Geometry check sheet. Reference: the model listing, model coordinates, mm. Coordinates: 2 decimals unless noted, no trailing zeros. Loops run counter-clockwise (first coordinate to the right, second up) from the corner with the lowest first, then second, coordinate; pieces in that order, holes last. Notation, with made-up numbers: (84.25, 63) - (117.25, 63) arc R19 ccw to (117.25, 73) - close; hole circle Ø4 at (68.25, 70.5). An arc over 180 degrees is marked (long way). One line per item, written item: value.
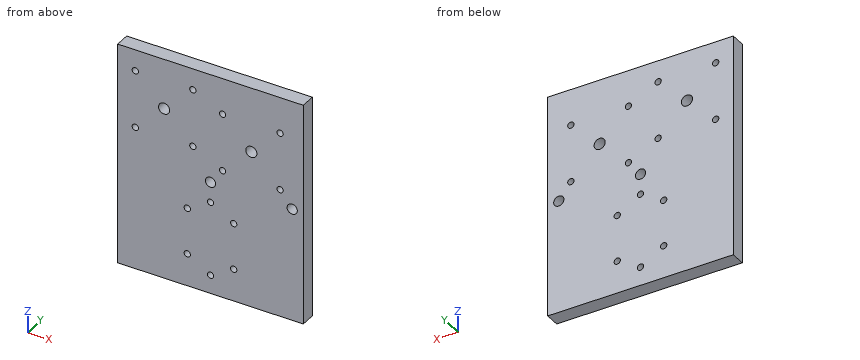
Autodesk Inventor part; units mm, degrees
ref_plane "YZ Plane" through (0, 0, 0) normal (1, 0, 0) x (0, 1, 0)
ref_plane "XZ Plane" through (0, 0, 0) normal (0, 1, 0) x (-1, 0, 0)
ref_plane "XY Plane" through (0, 0, 0) normal (0, 0, 1) x (1, 0, 0)
sketch "Skizze1" plane through (0, 0, 0) normal (0, 1, 0) x (-1, 0, 0)
  line L0 (50, -60) -> (-50, -60)
  line L1 (-50, -60) -> (-50, 60)
  line L2 (-50, 60) -> (50, 60)
  line L3 (50, 60) -> (50, -60)
  line L4 (50, -60) -> (-50, 60) construction
  line L5 (-50, -60) -> (50, 60) construction
  point P0 (0, 0)
  dimension "d0" = 100
  dimension "d1" = 120
extrude "Extrusion1" add sketch "Skizze1" along normal blind 8
sketch "Skizze2" plane through (0, 8, 0) normal (0, 1, 0) x (1, 0, 0)
  line L0 (-50, -60) -> (50, -60)
  line L1 (0, -60) -> (0, 152.9688)
  line L2 (50, 60) -> (-50, 60)
  point P0 (0, 0)
  point P1 (0, 10)
  point P2 (0, 50)
  dimension "d4" = 40
  dimension "d5" = 10
hole "Rail_through_holes" at (0, 8, -10) at (0, 8, -50) direction (0, -1, 0) diameter 3.4 end through all
sketch "Skizze3" plane through (0, 8, 0) normal (0, 1, 0) x (1, 0, 0)
  line L0 (-50, -60) -> (50, -60)
  line L1 (0, -60) -> (0, 60)
  line L2 (50, 60) -> (-50, 60)
  line L3 (12.5, 17.5) -> (-12.5, 17.5) construction
  line L4 (-12.5, 17.5) -> (-12.5, 42.5) construction
  line L5 (-12.5, 42.5) -> (12.5, 42.5) construction
  line L6 (12.5, 42.5) -> (12.5, 17.5) construction
  line L7 (12.5, 17.5) -> (-12.5, 42.5) construction
  line L8 (-12.5, 17.5) -> (12.5, 42.5) construction
  circle A0 centre (0, 50) radius 1.7 construction
  point P0 (0, 0)
  point P1 (0, 30)
  point P2 (0, 30)
  dimension "d13" = 25
  dimension "d14" = 25
  dimension "d15" = 20
hole "Slide_through_holes" at (-12.5, 8, -17.5) at (-12.5, 8, -42.5) at (12.5, 8, -42.5) at (12.5, 8, -17.5) direction (0, -1, 0) diameter 3.4 end through all
sketch "Skizze4" plane through (0, 8, 0) normal (0, 1, 0) x (1, 0, 0)
  line L0 (-50, -60) -> (50, -60)
  line L1 (0, -60) -> (0, 74.7934)
  line L2 (-25, -60) -> (-25, 181.0187) construction
  line L3 (-9.5, -48.5) -> (-40.5, -48.5) construction
  line L4 (-40.5, -48.5) -> (-40.5, -17.5) construction
  line L5 (-40.5, -17.5) -> (-9.5, -17.5) construction
  line L6 (-9.5, -17.5) -> (-9.5, -48.5) construction
  line L7 (-9.5, -48.5) -> (-40.5, -17.5) construction
  line L8 (-40.5, -48.5) -> (-9.5, -17.5) construction
  line L9 (50, 60) -> (-50, 60) construction
  circle A0 centre (-25, -33) radius 3
  point P0 (0, 0)
  point P1 (-25, -33)
  dimension "d23" = 25
  dimension "d24" = 31
  dimension "d25" = 31
  dimension "d26" = 93
  dimension "d60" = 6
hole "Nema_X_through_holes" at (-40.5, 8, 48.5) at (-40.5, 8, 17.5) at (-9.5, 8, 17.5) at (-9.5, 8, 48.5) direction (0, -1, 0) diameter 3.4 end through all
extrude "Nema_X_Shaft" cut sketch "Skizze4" against normal through all
sketch "Skizze5" plane through (0, 8, 0) normal (0, 1, 0) x (1, 0, 0)
  line L0 (-50, -60) -> (50, -60)
  line L1 (0, -60) -> (0, 63.3778)
  line L2 (22, -60) -> (22, 63.3778) construction
  line L3 (37.5, -40.5) -> (6.5, -40.5) construction
  line L4 (6.5, -40.5) -> (6.5, -9.5) construction
  line L5 (6.5, -9.5) -> (37.5, -9.5) construction
  line L6 (37.5, -9.5) -> (37.5, -40.5) construction
  line L7 (37.5, -40.5) -> (6.5, -9.5) construction
  line L8 (6.5, -40.5) -> (37.5, -9.5) construction
  circle A0 centre (22, -25) radius 3
  line L9 (50, 60) -> (-50, 60)
  line L10 (0, 88.0534) -> (0, -84.6756)
  point P0 (0, 0)
  point P1 (4.5, 5)
  point P2 (39.5, 5)
  point P3 (22, -25)
  dimension "d34" = 22
  dimension "d35" = 31
  dimension "d36" = 31
  dimension "d47" = 85
  dimension "d48" = 35
  dimension "d49" = 30
  dimension "d59" = 6
hole "Nema_Y_through_holes" at (6.5, 8, 40.5) at (6.5, 8, 9.5) at (37.5, 8, 9.5) at (37.5, 8, 40.5) direction (0, -1, 0) diameter 3.4 end through all
extrude "Nema_Y_Shaft" cut sketch "Skizze5" against normal through all
sketch "Skizze6" plane through (0, 8, 0) normal (0, 1, 0) x (1, 0, 0)
  circle A0 centre (22, -25) radius 3 construction
  line L0 (22, -25) -> (22, 60.1123) construction
  line L1 (0, 84) -> (0, -84) construction
  point P0 (0, 0)
  point P1 (0, -1)
  point P2 (44, -1)
  dimension "d50" = 44
  dimension "d51" = 24
hole "Y_Pulley_Shafts" at (0, 8, 1) at (44, 8, 1) direction (0, -1, 0) diameter 5.5 end through all
properties part number "14_XY_Plate" material "Aluminium 6061"
(1) Cross-section at B-B on x = -25. Record the cut outline in (y, z), and give its area (3 significant figures).
Reply:
outline: (0, -60) - (8, -60) - (8, 30) - (0, 30) - close; (0, 36) - (8, 36) - (8, 60) - (0, 60) - close
area: 912 mm2
(2) Cross-section at C-C on y = 5.5. State how many separate pieces and enclosed holes the cut face has, and give its area (3 significant figures).
Reply:
separate pieces: 1
enclosed holes: 18
area: 11,800 mm2
(3) Cross-section at D-D on x = 6.5. Record the cut outline in (y, z).
Reply:
outline: (0, -60) - (8, -60) - (8, 7.8) - (0, 7.8) - close; (0, 11.2) - (8, 11.2) - (8, 38.8) - (0, 38.8) - close; (0, 42.2) - (8, 42.2) - (8, 60) - (0, 60) - close
(4) Cross-section at A-A on z = 48.5. Record the cut outline in (x, y), and give its area (3 significant figures).
Reply:
outline: (-50, 0) - (-42.2, 0) - (-42.2, 8) - (-50, 8) - close; (-38.8, 0) - (-11.2, 0) - (-11.2, 8) - (-38.8, 8) - close; (-7.8, 0) - (50, 0) - (50, 8) - (-7.8, 8) - close
area: 746 mm2
(5) Material ranges on probe 1 along X at (y, z) = (4.5, 1); probe 2 along X at (y, z) = (2, 17.5); probe 3 along Z at (x, y) = (37.5, 4.5), recorded low to high. Write a range as from..to.
Reply:
probe 1: -50..-2.75, 2.75..41.25, 46.75..50
probe 2: -50..-42.2, -38.8..-11.2, -7.8..50
probe 3: -60..7.8, 11.2..38.8, 42.2..60
(6) Go/stop test with a flat-tipped pin: pin 1 Ø3 at (x, z) = (-12.5, -42.5) entering from +Y. Record where the tip stops, or that it passes through.
Reply:
pin 1: through
